Print and shaded views of the part. All mm, measured from the part's lowest x, y and z. A direction names the side the tool comes from. Round coordinates to 2 decimals unless told otherwise and drop trailing zeros. Loops run counter-clockwise (first coordinate to the right, second up) from the corner with the lowest first, then second, coordinate; pieces in that order, holes last. Notation, with made-up numbers: (26, 0) - (34, 0) arc R18 cw to (34, 13) - close; hole circle Ø10 at (-22, 72). An arc over 180 degrees is marked (long way). Answer as a JSON object with one key per item and string values.
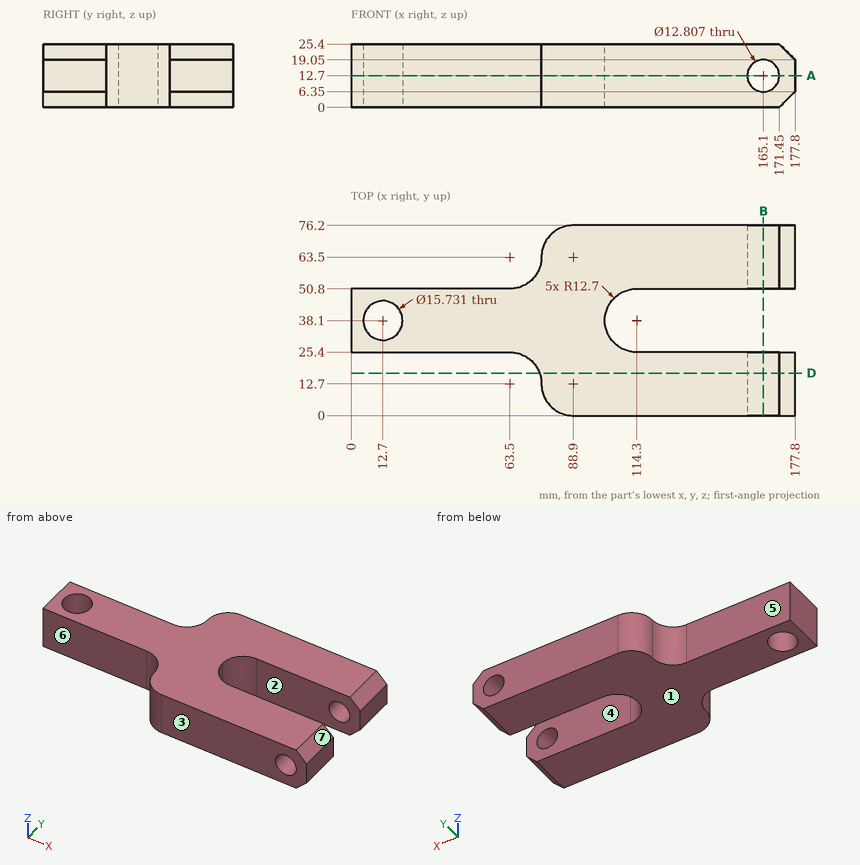
1) Drop flat-ended pins along their axis: P1, Ø12, axis at x = 32.5, z = 22.5, coming from the -Y side; P2, Ø4, axis at x = 64.5, z = 3.5, coming from the +Y side; P3, Ø5, axis at y = 44.5, z = 10.5, coming from the +X side. Give the stop position or say it passes through.
Values follow:
{"P1": "y = 25.4", "P2": "y = 51.16", "P3": "x = 105.24"}
2) Tool access for the marked faces 4, 5, 6 and 7: list every direction of +Z, -Z, +X, -X, +Y, -Y with a clear straight run to the whole face (end or side of a thin tool).
Values follow:
{"face 4": "+Z, -Z, +X", "face 5": "+Z, -Z, -X, +Y", "face 6": "+Z, -Z, -X, -Y", "face 7": "+Z, +X, +Y, -Y"}
3) Slice it at A-A on z = 12.7. List the corners of the cut face in (x, y) (1 decimal), then the cut area to 3 significant figures.
Values follow:
{"outline": "(0, 25.4) - (63.5, 25.4) arc R12.7 cw to (76.2, 12.7) arc R12.7 ccw to (88.9, 0) - (158.7, 0) - (158.7, 25.4) - (114.3, 25.4) arc R12.7 cw to (114.3, 50.8) - (158.7, 50.8) - (158.7, 76.2) - (88.9, 76.2) arc R12.7 ccw to (76.2, 63.5) arc R12.7 cw to (63.5, 50.8) - (0, 50.8) - close; (171.5, 0) - (177.8, 0) - (177.8, 25.4) - (171.5, 25.4) - close; (171.5, 50.8) - (177.8, 50.8) - (177.8, 76.2) - (171.5, 76.2) - close; hole circle Ø15.7 at (12.7, 38.1)", "area": "6,970 mm²"}
4) Slice it at B-B on x = 165.1. List the corners of the cut face in (y, z), then the cut area to 3 significant figures.
Values follow:
{"outline": "(0, 0) - (25.4, 0) - (25.4, 6.3) - (0, 6.3) - close; (0, 19.1) - (25.4, 19.1) - (25.4, 25.4) - (0, 25.4) - close; (50.8, 0) - (76.2, 0) - (76.2, 6.3) - (50.8, 6.3) - close; (50.8, 19.1) - (76.2, 19.1) - (76.2, 25.4) - (50.8, 25.4) - close", "area": "640 mm²"}
5) Probe probe 1 along Y at (x, z) = (12.7, 10.75) (1 decimal); probe 2 along Z at (x, y) = (165, 17); probe 3 along Y at (x, z) = (140, 15.5). List the from-to ranges inside material, lowest first.
Values follow:
{"probe 1": "25.4 to 30.2, 46 to 50.8", "probe 2": "0 to 6.3, 19.1 to 25.4", "probe 3": "0 to 25.4, 50.8 to 76.2"}
6) Two-plate mould, pull along Y, no slides. Class the marked faces 1, 2 and 3: pulls with the +Y half, pulls with the -Y half, needs draft (parallel to the pull), parting line crosses it, or undercut.
Values follow:
{"face 1": "needs draft", "face 2": "undercut", "face 3": "pulls with the -Y half"}
7) Slice it at D-D on y = 17. List the corners of the cut face in (x, z), then the cut area to 3 significant figures.
Values follow:
{"outline": "(75.45, 0) - (171.45, 0) - (177.8, 6.35) - (177.8, 19.05) - (171.45, 25.4) - (75.45, 25.4) - close; hole circle Ø12.81 at (165.1, 12.7)", "area": "2,430 mm²"}
